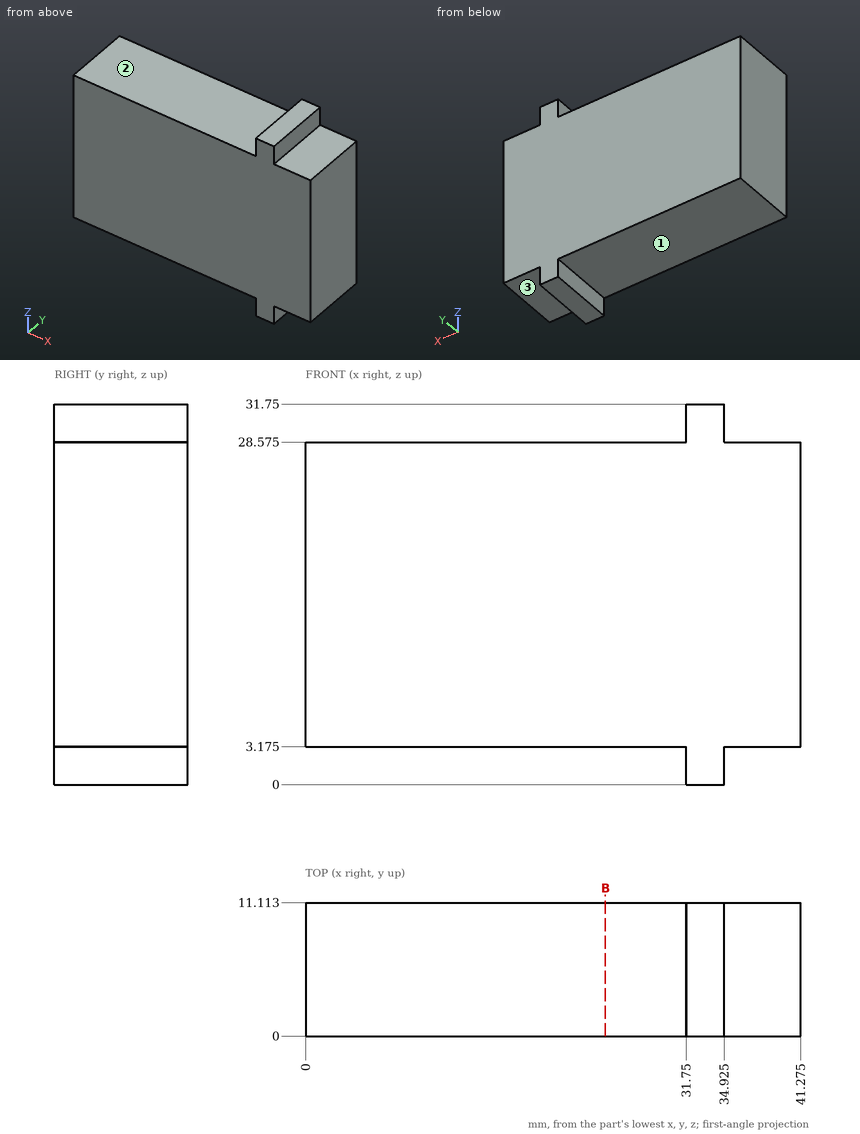
Source: three-view drawing plus pictorial views. Frame: mm from the lowest corner of the part. A direction names the side the tool comes from. Coordinates: 2 decimals unless noted, no trailing zeros. Order: outer loops, then holes, each group sorted by start corner. A loop starts at its lowest first (then second) coordinate and runs counter-clockwise, first axis right, second up. Notation, with made-up numbers: M 7.5,64.25 L 21.5,64.25 A18 cw 21.5,74.25 Z; hole C 36.5,66 d9. An arc over 180 degrees is marked long. Write each question's results on one line, items separated by ' | '. Start each with the question number.
1. Material intervals for L1, parallel to Z at x = 17, y = 1.5 (1 decimal), sorted ascending.
2. Reachability of the marked faces 1, 2 and 3 from +Z, -Z, +X, -X, +Y, -Y: full face, straight path, thin tool, end or side. Return the list, or none.
3. Pin query (flat end, axial travel): pin 1 (1 mm diameter, centred on x = 34, z = 25, fed in from -Y); pin 2 (1.6 mm diameter, centred on y = 6.5, z = 1.5, fed in from -X); pin 3 (5.5 mm diameter, centred on x = 10.5, y = 3, fed in from +Z) (1 decimal); pin 4 (5 mm diameter, centred on x = 37.5, y = 4.5, fed in from -Z) (1 decimal). Return the tip coordinate at first contact, or that it passes through.
4. Section B-B, the plane x = 25. Return the cut outline in (y, z) (1 decimal), then the cut area to 3 significant figures.
Solution:
1) L1: 3.2 to 28.6
2) face 1: -Z, -X, +Y, -Y | face 2: +Z, -X, +Y, -Y | face 3: -Z, +X, +Y, -Y
3) pin 1: y = 0 | pin 2: x = 31.75 | pin 3: z = 28.6 | pin 4: z = 3.2
4) outline: M 0,3.2 L 11.1,3.2 L 11.1,28.6 L 0,28.6 Z | area: 282 mm²
